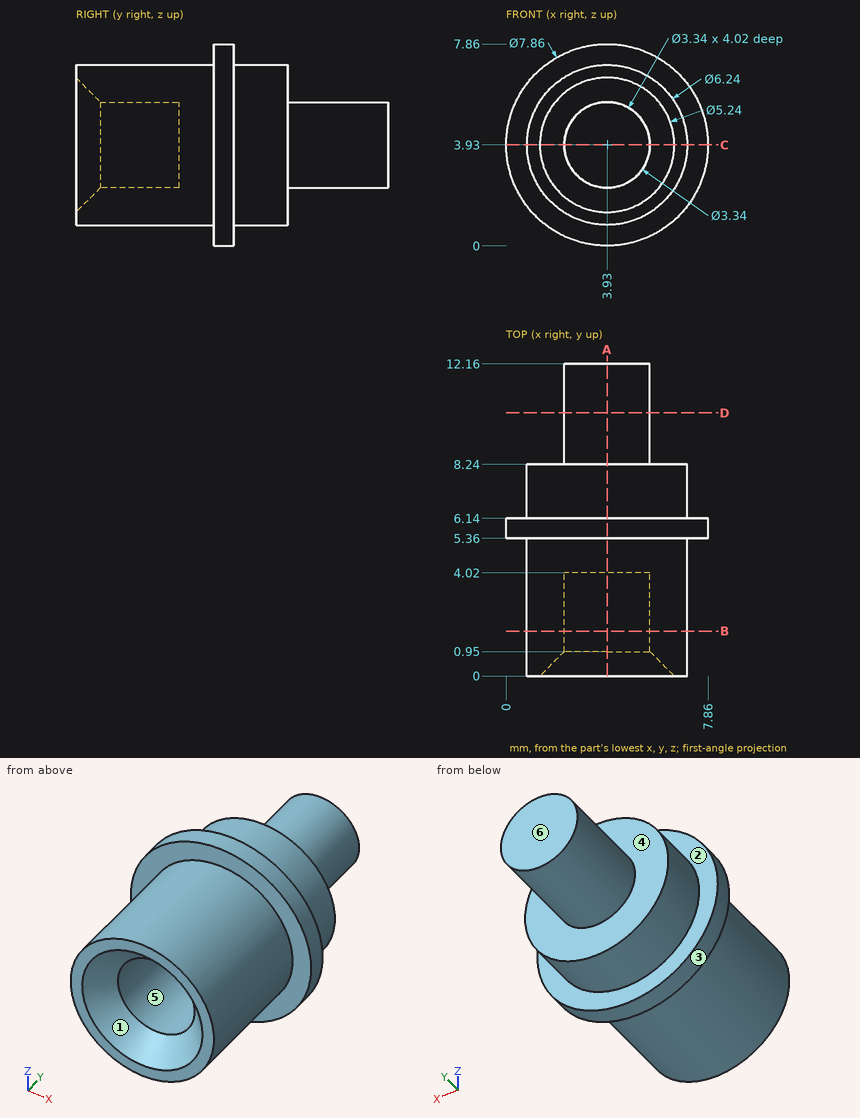
Source: three-view drawing plus pictorial views. Frame: mm from the lowest corner of the part. A direction names the side the tool comes from. Round coordinates to 2 decimals unless told otherwise and drop trailing zeros. Loops run counter-clockwise (first coordinate to the right, second up) from the corner with the lowest first, then second, coordinate; pieces in that order, holes last.
Q1. Section A-A on x = 3.93. Return loops of the section in (y, z), plus the area to 3 significant figures.
Q2. Material intervals for L1, parallel to X at y = 2.6, z = 3.93; L2, parallel to Y at x = 0.75, z = 6; L3, parallel to Y at x = 3.25, z = 3.25, sorted ascending.
Q3. Pull-direction query (Z, two-part tool) for the marked faces 1, 2 and 3; classes: released by +Z, released by -Z, zero draft, split by the parting line, or undercut.
Q4. Access query for the marked faces 4, 5 and 6. Directions: +Z, -Z, +X, -X, +Y, -Y. A direction counts if a zero-diameter tool reaches every point of the face in a straight line with its end or side. Return the directions, or none.
Q5. Section C-C on z = 3.93. Return loops of the section in (x, y).
Q6. Pin query (flat end, axial travel): P1, Ø4, axis at y = 10.5, z = 5, coming from the -X side; P2, Ø1.5, axis at y = 6, z = 2.5, coming from the -X side; P3, Ø3, axis at y = 2.5, z = 4, coming from the -X side. Return the tip coordinate at first contact, or that it passes through.
Q7. Section D-D on y = 10.25. Return loops of the section in (x, z), plus the area to 3 significant figures.
Q8. Section B-B on y = 1.75. Return loops of the section in (x, z), plus the area to 3 significant figures.
Evaluation:
1. outline: (0, 0.81) - (5.36, 0.81) - (5.36, 0) - (6.14, 0) - (6.14, 0.81) - (8.24, 0.81) - (8.24, 2.26) - (12.16, 2.26) - (12.16, 5.6) - (8.24, 5.6) - (8.24, 7.05) - (6.14, 7.05) - (6.14, 7.86) - (5.36, 7.86) - (5.36, 7.05) - (0, 7.05) - (0, 6.55) - (0.95, 5.6) - (4.02, 5.6) - (4.02, 2.26) - (0.95, 2.26) - (0, 1.31) - close
1. area: 51.4 mm2
2. L1: x = 0.81 to 2.26, 5.6 to 7.05
2. L2: y = 5.36 to 6.14
2. L3: y = 4.02 to 12.16
3. face 1: undercut
3. face 2: zero draft
3. face 3: split by the parting line
4. face 4: +Y
4. face 5: -Y
4. face 6: +Z, -Z, +X, -X, +Y
5. outline: (0, 5.36) - (0.81, 5.36) - (0.81, 0) - (1.31, 0) - (2.26, 0.95) - (2.26, 4.02) - (5.6, 4.02) - (5.6, 0.95) - (6.55, 0) - (7.05, 0) - (7.05, 5.36) - (7.86, 5.36) - (7.86, 6.14) - (7.05, 6.14) - (7.05, 8.24) - (5.6, 8.24) - (5.6, 12.16) - (2.26, 12.16) - (2.26, 8.24) - (0.81, 8.24) - (0.81, 6.14) - (0, 6.14) - close
6. P1: stops at x = 2.26
6. P2: stops at x = 0.06
6. P3: stops at x = 0.81
7. outline: circle Ø3.34 at (3.93, 3.93)
7. area: 8.76 mm2
8. outline: circle Ø6.24 at (3.93, 3.93); hole circle Ø3.34 at (3.93, 3.93)
8. area: 21.8 mm2
